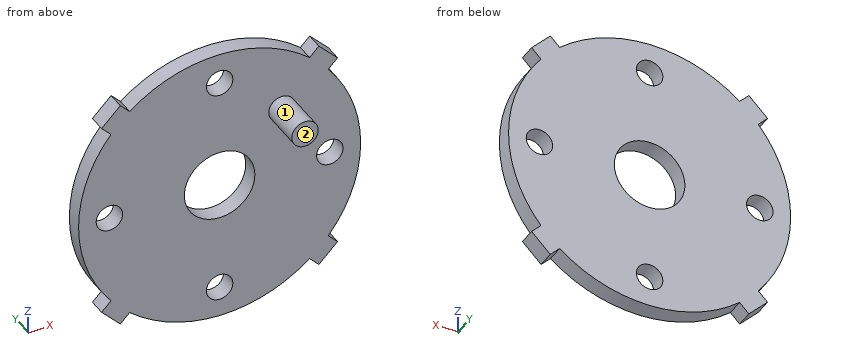
```python
from build123d import *

# Parameters (mm, degrees)
SKETCH1_R           = 16
SKETCH1_R_2         = 1.5
SKETCH1_R_3         = 4
BOSS_EXTRUDE1_DEPTH = 2
SKETCH2_R           = 1.5
BOSS_EXTRUDE2_DEPTH = 5


with BuildPart() as part:
    # Sketch1 → Boss-Extrude1 (new body)
    with BuildSketch(Plane(origin=(0, 0, 0), x_dir=(1, 0, 0), z_dir=(0, 1, 0))):
        Circle(SKETCH1_R)
        with Locations((-12.5, 0)):
            Circle(SKETCH1_R_2, mode=Mode.SUBTRACT)
        with Locations((0, -12.5)):
            Circle(SKETCH1_R_2, mode=Mode.SUBTRACT)
        with Locations((12.5, 0)):
            Circle(SKETCH1_R_2, mode=Mode.SUBTRACT)
        with Locations((0, 12.5)):
            Circle(SKETCH1_R_2, mode=Mode.SUBTRACT)
        Circle(SKETCH1_R_3, mode=Mode.SUBTRACT)
        with BuildLine():
            ThreePointArc((-10.203220154, -12.324540498), (-11.313708499, -11.313708499), (-12.324540498, -10.203220154))
            Line((-12.324540498, -10.203220154), (-13.38520067, -11.263880326))
            Line((-13.38520067, -11.263880326), (-11.263880326, -13.38520067))
            Line((-11.263880326, -13.38520067), (-10.203220154, -12.324540498))
        make_face()
        with BuildLine():
            Line((13.38520067, -11.263880326), (12.324540498, -10.203220154))
            ThreePointArc((12.324540498, -10.203220154), (11.313708499, -11.313708499), (10.203220154, -12.324540498))
            Line((10.203220154, -12.324540498), (11.263880326, -13.38520067))
            Line((11.263880326, -13.38520067), (13.38520067, -11.263880326))
        make_face()
        with BuildLine():
            Line((13.38520067, 11.263880326), (11.263880326, 13.38520067))
            Line((11.263880326, 13.38520067), (10.203220154, 12.324540498))
            ThreePointArc((10.203220154, 12.324540498), (11.313708499, 11.313708499), (12.324540498, 10.203220154))
            Line((12.324540498, 10.203220154), (13.38520067, 11.263880326))
        make_face()
        with BuildLine():
            ThreePointArc((-12.324540498, 10.203220154), (-11.313708499, 11.313708499), (-10.203220154, 12.324540498))
            Line((-10.203220154, 12.324540498), (-11.263880326, 13.38520067))
            Line((-11.263880326, 13.38520067), (-13.38520067, 11.263880326))
            Line((-13.38520067, 11.263880326), (-12.324540498, 10.203220154))
        make_face()
    extrude(amount=BOSS_EXTRUDE1_DEPTH)

    # Sketch2 → Boss-Extrude2 (add)
    with BuildSketch(Plane.XZ):
        with Locations((7.071067812, 7.071067812)):
            Circle(SKETCH2_R)
    extrude(amount=BOSS_EXTRUDE2_DEPTH)


solid = part.part
```
Can you work these out from the model? Positions are in its coordinate system, mm. Face numbers are marked on the shaded views. A direction names the side the tool comes from. Coordinates: 2 decimals unless noted, no trailing zeros. Loops run counter-clockwise (first coordinate to the right, second up) from the corner with the lowest first, then second, coordinate; pieces in that order, holes last. Notation, with made-up numbers: M 86.25,-27.75 L 131.25,-27.75 A24 cw 131.25,9.25 Z; hole C 68.5,-10 d1. An arc over 180 degrees is marked long. Put each result on its own line as item: value. Start each with the question number.
(1) I need wall thicknesses on probe 1 along X at (y, z) = (0.55, 0); probe 2 along Z at (x, y) = (-12.5, 0.5). Which ranges of each line are inside material? Lowest first, please.
(2) Imagine slicing it at C-C on z = -9. List the corners of the cut face in (x, y) for me.
(3) Will these pins go through, and if not, where does the flat tip stop? pin 1 Ø2 at (x, y) = (-6, 0.5) entering from +Z; pin 2 Ø8 at (x, z) = (-6, -7) entering from -Y.
(4) Imagine slicing it at A-A on x = 0. List the corners of the cut face in (y, z) for me, and give its area (3 significant figures).
(5) Imagine slicing it at B-B on z = 0. List the corners of the cut face in (x, y) for me, and give its area (3 significant figures).
(6) Imagine slicing it at D-D on y = -0.75. List the corners of the cut face in (x, z) for me, and give its area (3 significant figures).
(7) Which directions (+Z, -Z, +X, -X, +Y, -Y) give clear straight access to the entire face, cutting with the end or side of a thin tool? Please do the marked faces 1 and 2.
Worked answers:
1. probe 1: x = -16 to -14, -11 to -4, 4 to 11, 14 to 16
1. probe 2: z = -12.15 to -10.38, -9.99 to -1.5, 1.5 to 9.99, 10.38 to 12.15
2. outline: M -13.23,0 L 13.23,0 L 13.23,2 L -13.23,2 Z
3. pin 1: stops at z = 15.2
3. pin 2: stops at y = 0
4. outline: M 0,-16 L 2,-16 L 2,-14 L 0,-14 Z; M 0,-11 L 2,-11 L 2,-4 L 0,-4 Z; M 0,4 L 2,4 L 2,11 L 0,11 Z; M 0,14 L 2,14 L 2,16 L 0,16 Z
4. area: 36.0 mm2
5. outline: M -16,0 L -14,0 L -14,2 L -16,2 Z; M -11,0 L -4,0 L -4,2 L -11,2 Z; M 4,0 L 11,0 L 11,2 L 4,2 Z; M 14,0 L 16,0 L 16,2 L 14,2 Z
5. area: 36.0 mm2
6. outline: C 7.07,7.07 d3
6. area: 7.07 mm2
7. face 1: -Y
7. face 2: +Z, -Z, +X, -X, -Y
